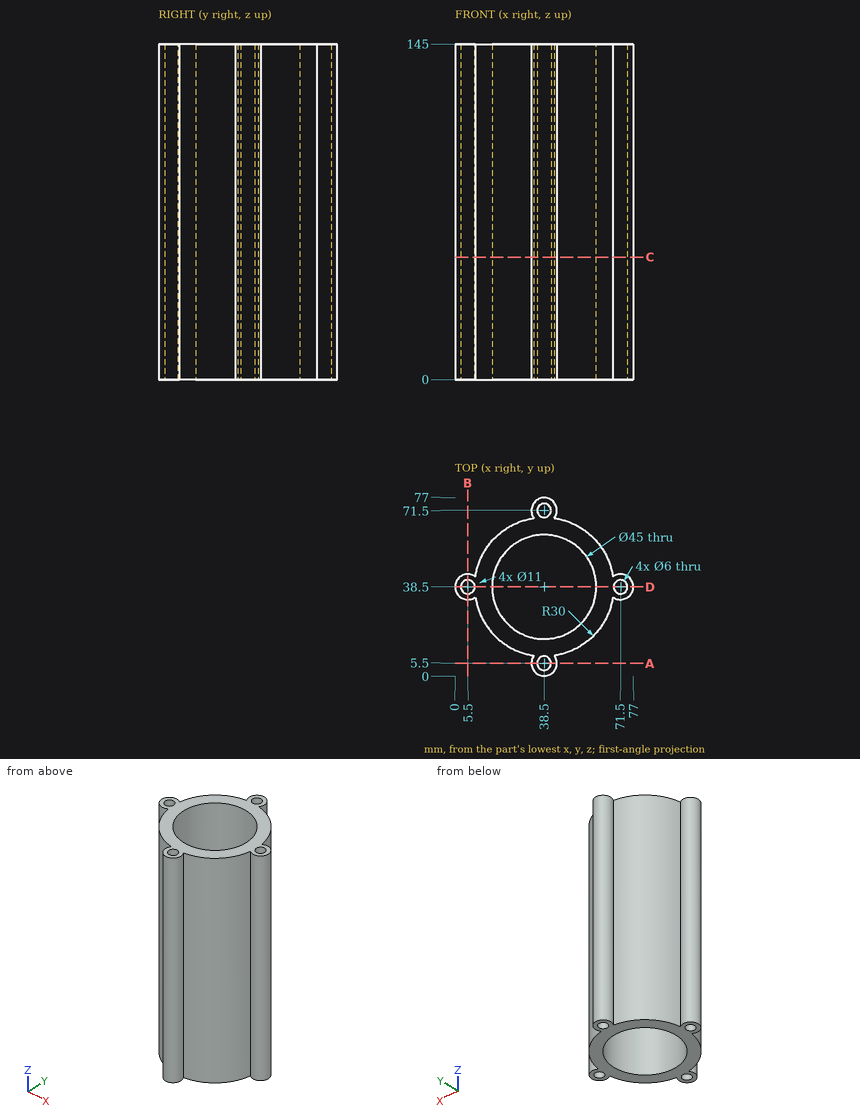
Drawing for the job (mm, zero at the part's lowest x, y, z). Round coordinates to 2 decimals unless told otherwise and drop trailing zeros. Loops run counter-clockwise (first coordinate to the right, second up) from the corner with the lowest first, then second, coordinate; pieces in that order, holes last. Notation, with made-up numbers: (-33, 11) -> (21, 11) arc R27 ccw to (21, 50) -> close; hole circle Ø4 at (-25, 55.25). An arc over 180 degrees is marked (long way). Answer as CSV lines item,"result". Start each with the question number.
1) Probe line 1 along X through (y, z) = (38, 109); line 2 along Y through (x, z) = (40.5, 8); line 3 along Y through (x, z) = (5.5, 79.5). List the from-to ranges inside material, lowest first.
2) Pin check, flat tips, straight feed: P1, Ø1.5, axis at y = 45.5, z = 15, coming from the -X side; P2, Ø10, axis at y = 61, z = 90.5, coming from the -X side; P3, Ø4, axis at y = 35, z = 75, coming from the +X side. Stop position of each tip, or through.
3) Slice it at D-D (y = 38.5). List the corners of the cut face in (x, z).
4) Slice it at C-C (z = 53). List the corners of the cut face in (x, y), plus the area to 3 significant figures.
5) Slice it at A-A (y = 5.5). List the corners of the cut face in (x, z), plus the area to 3 significant figures.
Filled in:
1,line 1,"x = 0.02 to 2.54, 8.46 to 16.01, 60.99 to 68.54, 74.46 to 76.98"
1,line 2,"y = 0.38 to 3.26, 7.74 to 16.09, 60.91 to 69.26, 73.74 to 76.62"
1,line 3,"y = 33 to 35.5, 41.5 to 44"
2,P1,"stops at x = 9.16"
2,P2,"stops at x = 14.13"
2,P3,"stops at x = 76.79"
3,outline,"(0, 0) -> (2.5, 0) -> (2.5, 145) -> (0, 145) -> close; (8.5, 0) -> (16, 0) -> (16, 145) -> (8.5, 145) -> close; (61, 0) -> (68.5, 0) -> (68.5, 145) -> (61, 145) -> close; (74.5, 0) -> (77, 0) -> (77, 145) -> (74.5, 145) -> close"
4,outline,"(8.82, 34.12) arc R30 ccw to (34.12, 8.82) arc R5.5 ccw (long way) to (42.88, 8.82) arc R30 ccw to (68.18, 34.12) arc R5.5 ccw (long way) to (68.18, 42.88) arc R30 ccw to (42.88, 68.18) arc R5.5 ccw (long way) to (34.12, 68.18) arc R30 ccw to (8.82, 42.88) arc R5.5 ccw (long way) to start; hole circle Ø6 at (5.5, 38.5); hole circle Ø45 at (38.5, 38.5); hole circle Ø6 at (38.5, 5.5); hole circle Ø6 at (38.5, 71.5); hole circle Ø6 at (71.5, 38.5)"
4,area,"1,440 mm2"
5,outline,"(33, 0) -> (35.5, 0) -> (35.5, 145) -> (33, 145) -> close; (41.5, 0) -> (44, 0) -> (44, 145) -> (41.5, 145) -> close"
5,area,"725 mm2"
